```python
from build123d import *

# Parameters (mm, degrees)
SZKIC1_R                    = 75
DODANIE_WYCI_GNI_CIE1_DEPTH = 40
SZKIC2_R                    = 6
WYTNIJ_WYCI_GNI_CIE1_DEPTH  = 40
SZKIC3_R                    = 47.5
WYTNIJ_WYCI_GNI_CIE2_DEPTH  = 40
SZKIC4_W                    = 50
SZKIC4_H                    = 20
DODANIE_WYCI_GNI_CIE2_DEPTH = 100
SZKIC6_W                    = 50
SZKIC6_H                    = 49.999779654
DODANIE_WYCI_GNI_CIE3_DEPTH = 20
SZKIC7_R                    = 7
WYTNIJ_WYCI_GNI_CIE3_DEPTH  = 226
ZAOKR_GLENIE1_R             = 24
ZAOKR_GLENIE2_R             = 10
DODANIE_WYCI_GNI_CIE4_DEPTH = 100
SZKIC10_W                   = 50
SZKIC10_H                   = 50
DODANIE_WYCI_GNI_CIE5_DEPTH = 100
SZKIC12_R                   = 7
WYTNIJ_WYCI_GNI_CIE5_DEPTH  = 163.5
WYTNIJ_WYCI_GNI_CIE6_DEPTH  = 161


with BuildPart() as part:
    # Szkic1 → Dodanie-wyciągnięcie1 (new body)
    with BuildSketch(Plane.XY):
        Circle(SZKIC1_R)
    extrude(amount=DODANIE_WYCI_GNI_CIE1_DEPTH)

    # Szkic2 → Wytnij-wyciągnięcie1 (cut)
    with BuildSketch(Plane.XY.offset(40)):
        with Locations((-55, 0)):
            Circle(SZKIC2_R)
        with Locations((0, 55)):
            Circle(SZKIC2_R)
        with Locations((55, 0)):
            Circle(SZKIC2_R)
        with Locations((0, -55)):
            Circle(SZKIC2_R)
    extrude(amount=-WYTNIJ_WYCI_GNI_CIE1_DEPTH, mode=Mode.SUBTRACT)

    # Szkic3 → Wytnij-wyciągnięcie2 (cut)
    with BuildSketch(Plane.XY.offset(40)):
        Circle(SZKIC3_R)
    extrude(amount=-WYTNIJ_WYCI_GNI_CIE2_DEPTH, mode=Mode.SUBTRACT)

    # Szkic4 → Dodanie-wyciągnięcie2 (add, symmetric)
    with BuildSketch(Plane(origin=(0, 0, 0), x_dir=(-0.707106781, -0.707106781, 0), z_dir=(0.707106781, -0.707106781, 0))):
        with Locations((0, 10)):
            Rectangle(SZKIC4_W, SZKIC4_H)
    extrude(amount=DODANIE_WYCI_GNI_CIE2_DEPTH, both=True)

    # Szkic6 → Dodanie-wyciągnięcie3 (add)
    with BuildSketch(Plane(origin=(70.710678119, -70.710678119, 0), x_dir=(0, 0, -1), z_dir=(0.707106781, -0.707106781, 0))):
        with Locations((45, 0.000110173)):
            Rectangle(SZKIC6_W, SZKIC6_H)
    dodanie_wyci_gni_cie3 = extrude(amount=-DODANIE_WYCI_GNI_CIE3_DEPTH)

    # Lustro1: Dodanie-wyciągnięcie3 across plane
    add(dodanie_wyci_gni_cie3.mirror(Plane(origin=(0, 0, 0), x_dir=(0, 0, 1), z_dir=(0.707106781, -0.707106781, 0))))

    # Szkic7 → Wytnij-wyciągnięcie3 (cut, through all)
    with BuildSketch(Plane(origin=(-70.710678119, 70.710678119, 0), x_dir=(0, 0, 1), z_dir=(-0.707106781, 0.707106781, 0))):
        with Locations((-45, 0)):
            Circle(SZKIC7_R)
    extrude(amount=-WYTNIJ_WYCI_GNI_CIE3_DEPTH, mode=Mode.SUBTRACT)

    # Zaokrąglenie1
    zaokr_glenie1_edges = [part.edges().sort_by_distance(p)[0] for p in [
        (81.317279836, -45.961940777, -70),
        (45.962096585, -81.317124028, -70),
        (-81.317124028, 45.962096585, -70),
        (-45.961940777, 81.317279836, -70),
    ]]
    fillet(zaokr_glenie1_edges, radius=ZAOKR_GLENIE1_R)

    # Zaokrąglenie2
    zaokr_glenie2_edges = [part.edges().sort_by_distance(p)[0] for p in [
        (-70.710678119, 70.710678119, 0),
        (70.710678119, -70.710678119, 0),
    ]]
    fillet(zaokr_glenie2_edges, radius=ZAOKR_GLENIE2_R)

    # Szkic8 → Dodanie-wyciągnięcie4 (add)
    with BuildSketch(Plane(origin=(0, 0, -20), x_dir=(-1, 0, 0), z_dir=(0, 0, -1))):
        Polygon((0, 35.355339059), (35.355339059, 0), (0, -35.355339059), (-35.355339059, 0), align=None)
    extrude(amount=DODANIE_WYCI_GNI_CIE4_DEPTH)

    # Szkic10 → Dodanie-wyciągnięcie5 (add)
    with BuildSketch(Plane(origin=(17.67766953, 17.67766953, 0), x_dir=(0, 0, -1), z_dir=(0.707106781, 0.707106781, 0))):
        with Locations((95, 0)):
            Rectangle(SZKIC10_W, SZKIC10_H)
    extrude(amount=DODANIE_WYCI_GNI_CIE5_DEPTH)

    # Szkic12 → Wytnij-wyciągnięcie5 (cut, through all)
    with BuildSketch(Plane(origin=(17.67766953, -17.67766953, 0), x_dir=(0, 0, -1), z_dir=(0.707106781, -0.707106781, 0))):
        with Locations((95, 105)):
            Circle(SZKIC12_R)
    extrude(amount=-WYTNIJ_WYCI_GNI_CIE5_DEPTH, mode=Mode.SUBTRACT)

    # Szkic14 → Wytnij-wyciągnięcie6 (cut, through all)
    with BuildSketch(Plane(origin=(0, 0, -120), x_dir=(-1, 0, 0), z_dir=(0, 0, -1))):
        with BuildLine():
            Line((-80.610173055, 60.811183182), (-98.287842585, 78.488852712))
            Line((-98.287842585, 78.488852712), (-78.488852712, 98.287842585))
            Line((-78.488852712, 98.287842585), (-60.811183182, 80.610173055))
            ThreePointArc((-60.811183182, 80.610173055), (-60.811183182, 60.811183182), (-80.610173055, 60.811183182))
        make_face()
    extrude(amount=-WYTNIJ_WYCI_GNI_CIE6_DEPTH, mode=Mode.SUBTRACT)


solid = part.part
```
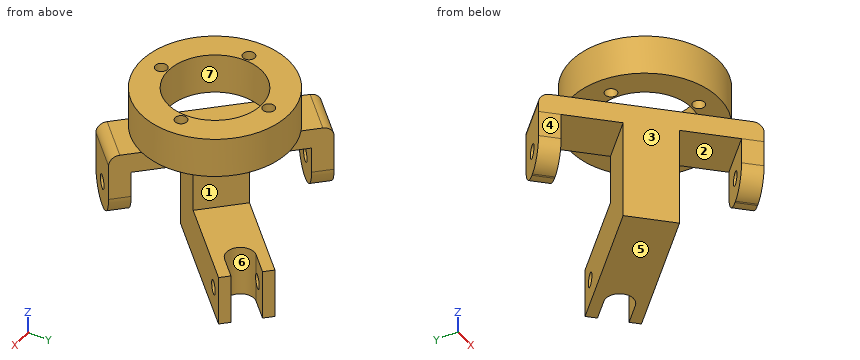
Check sheet for the modelled part. Datum: model origin and axes. Units: mm. Face numbers are marked on the shaded views. A direction names the side the tool comes from. Coordinates: 2 decimals unless noted, no trailing zeros. Loops run counter-clockwise (first coordinate to the right, second up) from the corner with the lowest first, then second, coordinate; pieces in that order, holes last. Notation, with made-up numbers: M -38.5,43.25 L -22.5,43.25 A31 cw -22.5,68.25 Z; hole C -3,-30 d11. An arc over 180 degrees is marked long. Answer as a JSON object with one key per item and string values.
1. Release check for a two-part mould opening along Y. For the marked faces 4, 5, 6 and 7 record: pulls with the +Y half, pulls with the -Y half, needs draft (parallel to the pull), parting line crosses it, or undercut.
Outcome:
{"face 4": "pulls with the -Y half", "face 5": "needs draft", "face 6": "undercut", "face 7": "undercut"}
2. Sectioned sample at C-C on z = -60. Record the cut outline in (x, y), and give its area (3 significant figures).
Outcome:
{"outline": "M -85.2,56.22 L -71.06,42.08 L -42.08,71.06 L -56.22,85.2 Z; M -35.36,0 L 0,-35.36 L 35.36,0 L 0,35.36 Z; M 42.08,-71.06 L 56.22,-85.2 L 85.2,-56.22 L 71.06,-42.08 Z", "area": "4,140 mm²"}
3. Depth check by flat-ended pin: P1, Ø22.5, axis at x = 47, y = -65, coming from the -Z side; P2, Ø8, axis at x = -43, y = 12, coming from the -Z side; P3, Ø3, axis at x = 65, y = 54.5, coming from the +Z side. Enter the tip coordinate at first touch or a pass-through.
Outcome:
{"P1": "z = -69.99", "P2": "z = -20", "P3": "z = -70"}
4. Sectioned sample at A-A on z = -30. Record the cut outline in (x, y), and give its area (3 significant figures).
Outcome:
{"outline": "M -88.39,53.03 L -74.25,38.89 L -38.89,74.25 L -53.03,88.39 Z; M -35.36,0 L 0,-35.36 L 35.36,0 L 0,35.36 Z; M 38.89,-74.25 L 53.03,-88.39 L 88.39,-53.03 L 74.25,-38.89 Z", "area": "4,500 mm²"}
5. Scan lines: L1, parallel to Y at x = 0, z = 20.5; L2, parallel to Z at x = -13.5, y = 42.5; L3, parallel to Z at x = 23, y = 44.5. Record each from-to range of solid material in increasing order. Write a range as from..to.
Outcome:
{"L1": "-75..-61, -49..-47.5, 47.5..49, 61..75", "L2": "-20..0", "L3": "-120..-70, 0..40"}
6. Sectioned sample at B-B on x = -18.5. Record the cut outline in (y, z), and give its area (3 significant figures).
Outcome:
{"outline": "M -72.68,0 L -43.75,0 L -43.75,40 L -72.68,40 Z; M -16.86,-120 L 16.86,-120 L 16.86,-20 L 53.86,-20 L 53.86,0 L 72.68,0 L 72.68,40 L 43.75,40 L 43.75,0 L -16.86,0 Z", "area": "7,100 mm²"}
7. Access from +Z, -Z, +X, -X, +Y, -Y to the whole of each face (thin tool, end or side, straight path). Record for the marked faces 1, 2 and 3.
Outcome:
{"face 1": "+X, +Y", "face 2": "-Z", "face 3": "-Z, -X, -Y"}
